Verification items for the finished model (mm, model axes). Face numbers are marked on the shaded views. Round coordinates to 2 decimals unless told otherwise and drop trailing zeros. Write each loop counter-clockwise with the first axis right and the second up, starting at its lowest first coordinate (ties: lowest second). Pieces come first, ordered by that corner, then holes.
from build123d import *

# Parameters (mm, degrees)
SKETCH1_R           = 1.65
BOSS_EXTRUDE1_DEPTH = 5
SKETCH2_R           = 1.65
CUT_EXTRUDE1_DEPTH  = 5
CHAMFER1_SIZE       = 2
CHAMFER1_SIZE2      = 1.154700538
SKETCH3_W           = 1.5
SKETCH3_H           = 2
CUT_EXTRUDE2_DEPTH  = 47.5


with BuildPart() as part:
    # Sketch1 → Boss-Extrude1 (new body)
    with BuildSketch(Plane.XY):
        with BuildLine():
            Line((0, 5), (35, 5))
            ThreePointArc((35, 5), (40, 0), (35, -5))
            Line((35, -5), (0, -5))
            ThreePointArc((0, -5), (-5, 0), (0, 5))
        make_face()
        with Locations((35, 0)):
            Circle(SKETCH1_R, mode=Mode.SUBTRACT)
        Circle(SKETCH1_R, mode=Mode.SUBTRACT)
    extrude(amount=BOSS_EXTRUDE1_DEPTH)

    # Sketch2 → Cut-Extrude1 (cut)
    with BuildSketch(Plane.XY.offset(5)):
        with Locations((17.5, 0)):
            Circle(SKETCH2_R)
    extrude(amount=-CUT_EXTRUDE1_DEPTH, mode=Mode.SUBTRACT)

    # Chamfer1
    chamfer1_edges = [part.edges().sort_by_distance(p)[0] for p in [
        (15.85, 0, 5),
    ]]
    chamfer1_side = [part.faces().sort_by_distance(p)[0] for p in [
        (17.5, 4.539022777, 5),
    ]]
    chamfer(chamfer1_edges, length=CHAMFER1_SIZE, length2=CHAMFER1_SIZE2, reference=chamfer1_side[0])

    # Sketch3 → Cut-Extrude2 (cut, symmetric)
    with BuildSketch(Plane(origin=(0, 0, 0), x_dir=(0, 0, -1), z_dir=(1, 0, 0))):
        with Locations((-4.25, 4)):
            Rectangle(SKETCH3_W, SKETCH3_H)
    extrude(amount=CUT_EXTRUDE2_DEPTH, both=True, mode=Mode.SUBTRACT)


solid = part.part
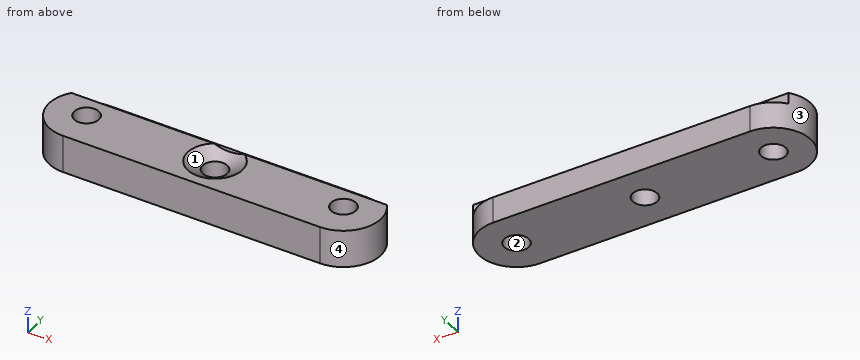
Q1. Material ranges on line 1 along Y through (x, z) = (17.5, 2.9); line 2 along X through (y, z) = (-0.75, 3.4); line 3 along X through (y, z) = (1, 0.8), recorded low to high.
Recorded:
line 1: y = -5 to -1.65, 1.65 to 5
line 2: x = -4.94 to -1.47, 1.47 to 16.03, 18.97 to 33.53, 36.47 to 39.94
line 3: x = -4.9 to -1.31, 1.31 to 16.19, 18.81 to 33.69, 36.31 to 39.9
Q2. Sectioned sample at C-C (x = 17.5). Enter the section's corners in (y, z), plus the area to 3 significant figures.
Recorded:
outline: (-5, 0) - (-1.65, 0) - (-1.65, 3.85) - (-3.65, 5) - (-5, 5) - close; (1.65, 0) - (5, 0) - (5, 3.5) - (3, 3.5) - (3, 4.62) - (1.65, 3.85) - close
area: 28.3 mm2
Q3. Sectioned sample at D-D (x = 5). Enter the section's corners in (y, z), plus the area to 3 significant figures.
Recorded:
outline: (-5, 0) - (5, 0) - (5, 3.5) - (3, 3.5) - (3, 5) - (-5, 5) - close
area: 47.0 mm2
Q4. Sectioned sample at A-A (y = 0). Enter the section's corners in (x, z), plus the area to 3 significant figures.
Recorded:
outline: (-5, 0) - (-1.65, 0) - (-1.65, 5) - (-5, 5) - close; (1.65, 0) - (15.85, 0) - (15.85, 3.85) - (13.85, 5) - (1.65, 5) - close; (19.15, 0) - (33.35, 0) - (33.35, 5) - (21.15, 5) - (19.15, 3.85) - close; (36.65, 0) - (40, 0) - (40, 5) - (36.65, 5) - close
area: 173 mm2
Q5. Depth check by flat-ended pin: P1, Ø1.5, axis at y = 3, z = 2.5, coming from the +X side; P2, Ø2.5, axis at x = 17.5, y = 0, coming from the +Z side; P3, Ø0.8, axis at x = 8, z = 4, coming from the +Y side; P4, Ø0.6, axis at x = 11, y = 4, coming from the +Z side. Enter the tip coordinate at first touch or a pass-through.
Recorded:
P1: stops at x = 39.47
P2: passes through
P3: stops at y = 3
P4: stops at z = 3.5
Q6. Sectioned sample at B-B (z = 2.65). Enter the section's corners in (x, y).
Recorded:
outline: (0, -5) - (35, -5) arc R5 ccw to (35, 5) - (0, 5) arc R5 ccw to start; hole circle Ø3.3 at (0, 0); hole circle Ø3.3 at (17.5, 0); hole circle Ø3.3 at (35, 0)
Q7. Release check for a two-part mould opening along X. For the marked faces 1, 2, 3 and 4 record: released by +X, released by -X, zero draft, split by the parting line, or undercut.
Recorded:
face 1: undercut
face 2: undercut
face 3: released by -X
face 4: released by +X
